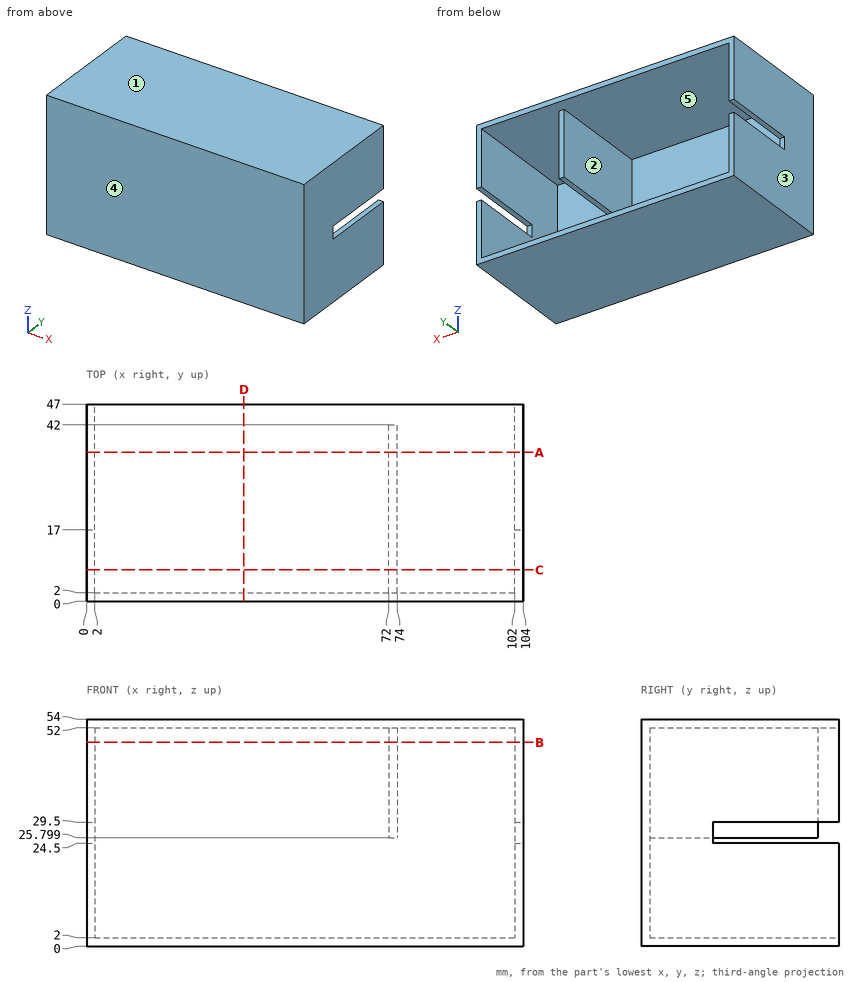
Input: dimensioned drawing with shaded views. Units: mm. Origin: part minimum x, y, z. A direction names the side the tool comes from. Coordinates: 2 decimals unless noted, no trailing zeros. Loops run counter-clockwise (first coordinate to the right, second up) from the corner with the lowest first, then second, coordinate; pieces in that order, holes last. Notation, with made-up numbers: M -26.75,18.25 L 3.25,18.25 A19 ccw 3.25,30.25 Z; hole C 58,77.25 d9. An arc over 180 degrees is marked long. One line per item, written item: value.
(1) Section C-C (y = 7.5). Output: boundary loops of the cut face in (x, z).
Filled in:
outline: M 0,0 L 104,0 L 104,54 L 0,54 Z; hole M 2,2 L 102,2 L 102,52 L 74,52 L 74,25.8 L 72,25.8 L 72,52 L 2,52 Z
(2) Line query: line 1 along X through (y, z) = (27.5, 48.5); line 2 along X through (y, z) = (45.5, 50); line 3 along Z through (x, y) = (41.5, 16). Output: solid intervals per line, ascending. Write a range as from..to.
Filled in:
line 1: 0..2, 72..74, 102..104
line 2: 0..2, 102..104
line 3: 0..2, 52..54
(3) Pin query (flat end, axial travel): pin 1 (13 mm diameter, centred on y = 21, z = 44.5, fed in from -X); pin 2 (2 mm diameter, centred on y = 19.5, z = 26.5, fed in from +X); pin 3 (2 mm diameter, centred on x = 0.5, z = 26, fed in from +Y); pin 4 (1 mm diameter, centred on x = 72.5, z = 36.5, fed in from +Y). Return the tip coordinate at first contact, or that it passes through.
Filled in:
pin 1: x = 0
pin 2: x = 74
pin 3: y = 17
pin 4: y = 42
(4) Section B-B (z = 48.5). Output: boundary loops of the cut face in (x, y), and give its area (3 significant figures).
Filled in:
outline: M 0,0 L 104,0 L 104,47 L 102,47 L 102,2 L 74,2 L 74,42 L 72,42 L 72,2 L 2,2 L 2,47 L 0,47 Z
area: 468 mm^2
(5) Section D-D (x = 37.5). Output: boundary loops of the cut face in (y, z).
Filled in:
outline: M 0,0 L 47,0 L 47,2 L 2,2 L 2,52 L 47,52 L 47,54 L 0,54 Z
(6) Section A-A (y = 35.5). Output: boundary loops of the cut face in (x, z).
Filled in:
outline: M 0,0 L 104,0 L 104,24.5 L 102,24.5 L 102,2 L 2,2 L 2,24.5 L 0,24.5 Z; M 0,29.5 L 2,29.5 L 2,52 L 72,52 L 72,25.8 L 74,25.8 L 74,52 L 102,52 L 102,29.5 L 104,29.5 L 104,54 L 0,54 Z
(7) Pull-direction query (X, two-part tool) for the marked faces 1, 2 and 3; classes: +X half, -X half, draft (parallel to the pull), parting line (faces both ways), or undercut.
Filled in:
face 1: draft
face 2: undercut
face 3: -X half
(8) Reachability of the marked faces 4 and 5 from +Z, -Z, +X, -X, +Y, -Y: full face, straight path, thin tool, end or side. Return the list, or none.
Filled in:
face 4: +Z, -Z, +X, -X, -Y
face 5: +Y
